```python
from build123d import *

# Parameters (mm, degrees)
SKETCH1_R           = 34.11
SKETCH1_R_2         = 31.75
BOSS_EXTRUDE1_DEPTH = 9.4
CUT_EXTRUDE1_DEPTH  = 69.22
CIRPATTERN2_COUNT   = 2
CIRPATTERN2_ANGLE   = 90


with BuildPart() as part:
    # Sketch1 → Boss-Extrude1 (new body)
    with BuildSketch(Plane.XY):
        Circle(SKETCH1_R)
        Circle(SKETCH1_R_2, mode=Mode.SUBTRACT)
    extrude(amount=BOSS_EXTRUDE1_DEPTH)

    # Sketch2 → Cut-Extrude1 (cut, through all)
    with BuildSketch(Plane(origin=(0, 34.11, 0), x_dir=(1, 0, 0), z_dir=(0, 1, 0))):
        Polygon((3.92598183, -5), (1.962990915, -1.6), (-1.962990915, -1.6), (-3.92598183, -5), (-1.962990915, -8.4), (1.962990915, -8.4), align=None)
    cut_extrude1 = extrude(amount=-CUT_EXTRUDE1_DEPTH, mode=Mode.SUBTRACT)

    # CirPattern2: Cut-Extrude1 ×2 about axis
    cirpattern2_axis = Axis((0, 0, 9.4), (0, 0, 1))
    for i in range(1, CIRPATTERN2_COUNT):
        add(cut_extrude1.rotate(cirpattern2_axis, i * CIRPATTERN2_ANGLE / (CIRPATTERN2_COUNT - 1)), mode=Mode.SUBTRACT)


solid = part.part
```
For this review, take the finished solid that the model builds, in its own axes (mm). A direction names the side the tool comes from. Coordinates: 2 decimals unless noted, no trailing zeros. Loops run counter-clockwise (first coordinate to the right, second up) from the corner with the lowest first, then second, coordinate; pieces in that order, holes last.
1. For faces 1 (the cylindrical face through (30.284, 9.537, 4.634)), 2 (the flat face through (-33, 0, 1.6)), 3 (the flat face through (2.931, -32.762, 6.724)), list the 3-axis set-ups (+Z, -Z, +X, -X, +Y, -Y) from which the entire face can be reached by the end or side of a thin tool; tool diameter is ignored.
2. For line 1 (X direction, y = 5.5, z = 4.5); line 2 (Y direction, x = 25.5, z = 3.5); line 3 (Y direction, x = -22, z = 1.25), list the stretches that pass through material, from the lowest coordinate up.
3. Add section D-D, the plane y = -19. Give the boundary of the cut face in (x, z), then the cut area to 3 significant figures.
4. Insertion check: P1, Ø4, axis at x = -20.5, z = 5, coming from the -Y side; P2, Ø4, axis at x = 18, z = 3.5, coming from the -Y side; P3, Ø5, axis at y = 24.5, z = 4, coming from the -X side. Each pin has a flat end and moves straight along its axis. Give the tip position at first contact, or say it passes through.
5. Add section C-C, the plane x = -13. Give the boundary of the cut face in (y, z).
6. Add section A-A, the plane y = 0. Give the boundary of the cut face in (x, z), then the cut area to 3 significant figures.
7. Mouldability with a two-part tool opening along X and no side actions: class faces 4 (the flat face through (0, -33, 1.6)), 5 (the flat face through (0, 33, 8.4)), 6 (the flat face through (-32.798, 2.931, 6.724)) as +X half, -X half, draft (parallel to the pull), parting line (faces both ways), or undercut.
Result:
1. face 1: +Z, -Z
1. face 2: +X, -X
1. face 3: +Y, -Y
2. line 1: x = -33.66 to -31.27, 31.27 to 33.66
2. line 2: y = -22.65 to -18.92, 18.92 to 22.65
2. line 3: y = -26.07 to -22.89, 22.89 to 26.07
3. outline: (-28.33, 0) - (-25.44, 0) - (-25.44, 9.4) - (-28.33, 9.4) - close; (25.44, 0) - (28.33, 0) - (28.33, 9.4) - (25.44, 9.4) - close
3. area: 54.3 mm2
4. P1: stops at y = -28.66
4. P2: stops at y = -30.12
4. P3: stops at x = -26.07
5. outline: (-31.54, 0) - (-28.97, 0) - (-28.97, 9.4) - (-31.54, 9.4) - close; (28.97, 0) - (31.54, 0) - (31.54, 9.4) - (28.97, 9.4) - close
6. outline: (-34.11, 0) - (-31.75, 0) - (-31.75, 1.6) - (-34.11, 1.6) - close; (-34.11, 8.4) - (-31.75, 8.4) - (-31.75, 9.4) - (-34.11, 9.4) - close; (31.75, 0) - (34.11, 0) - (34.11, 1.6) - (31.75, 1.6) - close; (31.75, 8.4) - (34.11, 8.4) - (34.11, 9.4) - (31.75, 9.4) - close
6. area: 12.3 mm2
7. face 4: undercut
7. face 5: undercut
7. face 6: draft
